CAD build for the part. Positions are in the model's coordinates, mm. A direction names the side the tool comes from. Give positions to 0.01 mm unless a question says otherwise; leave off trailing zeros. Order: outer loops, then holes, each group sorted by start corner. A loop starts at its lowest first (then second) coordinate and runs counter-clockwise, first axis right, second up.
```python
from build123d import *

# Parameters (mm, degrees)
BOSS_EXTRUDE1_DEPTH           = 45
SKETCH3_W                     = 30
SKETCH3_H                     = 40
CUT_EXTRUDE1_DEPTH            = 88.304481557
SKETCH4_W                     = 32
SKETCH4_H                     = 32
SKETCH4_W_2                   = 20.5
SKETCH4_H_2                   = 20.5
BOSS_EXTRUDE2_DEPTH           = 35
SKETCH6_W                     = 5
SKETCH6_H                     = 5
CUT_EXTRUDE4_DEPTH            = 35
RIB1_REACH                    = 87.394
SKETCH9_WALL_W                = 221.994100462
SKETCH9_WALL_H                = 2
LPATTERN1_COUNT               = 2
LPATTERN1_PITCH               = 20
RIB6_REACH                    = 100.659
SKETCH14_WALL_W               = 234.916193708
SKETCH14_WALL_H               = 2
RIB7_START                    = -2
RIB7_DEPTH                    = 2
FILLET2_R                     = 5
FILLET3_R                     = 5
RIB10_REACH                   = 92.525
SKETCH17_WALL_W               = 226.71130823
SKETCH17_WALL_H               = 2
RIB11_REACH                   = 92.525
SKETCH18_WALL_W               = 226.71130823
SKETCH18_WALL_H               = 2
FILLET4_R                     = 10
LPATTERN2_COUNT               = 2
LPATTERN2_PITCH               = 43
FILLET4_OF_LPATTERN2_R        = 10
M5_CLEARANCE_HOLE2_AT_2_COUNT = 2
M5_CLEARANCE_HOLE2_AT_2_PITCH = 15
M2_5_CLEARANCE_HOLE1_D        = 2.9
FILLET5_R                     = 2.5
SKETCH4_4_R                   = 2.5
BOSS_EXTRUDE4_DEPTH           = 8
CIRPATTERN1_COUNT             = 4


# Read off the part's stored shape, not the designer's step: Rib7
with BuildPart() as part:
    # Sketch2 → Boss-Extrude1 (new body)
    with BuildSketch(Plane.XY):
        Polygon((-53.5125, -22.5), (17.8375, -22.5), (17.8375, -17.5), (-8.5125, -17.5), (-8.5125, 22.5), (-13.5125, 22.5), (-13.5125, -17.5), (-48.5125, -17.5), (-48.5125, 22.5), (-53.5125, 22.5), align=None)
    extrude(amount=BOSS_EXTRUDE1_DEPTH)

    # Sketch3 → Cut-Extrude1 (cut, through all)
    with BuildSketch(Plane(origin=(-53.5125, 0, 0), x_dir=(0, 0, -1), z_dir=(1, 0, 0))):
        with Locations((-22.5, 2.5)):
            Rectangle(SKETCH3_W, SKETCH3_H)
    extrude(amount=CUT_EXTRUDE1_DEPTH, mode=Mode.SUBTRACT)

    # Sketch4 → Boss-Extrude2 (add)
    with BuildSketch(Plane.XZ.offset(22.5)):
        with Locations((1.8375, 22.5)):
            Rectangle(SKETCH4_W, SKETCH4_H)
        with Locations((1.8375, 22.5)):
            Rectangle(SKETCH4_W_2, SKETCH4_H_2, mode=Mode.SUBTRACT)
    extrude(amount=BOSS_EXTRUDE2_DEPTH)

    # Sketch6 → Cut-Extrude4 (cut)
    with BuildSketch(Plane(origin=(0, -57.5, 0), x_dir=(-1, 0, 0), z_dir=(0, -1, 0))):
        with Locations((11.6625, -36)):
            Rectangle(SKETCH6_W, SKETCH6_H)
        with Locations((-15.3375, -36)):
            Rectangle(SKETCH6_W, SKETCH6_H)
        with Locations((-15.3375, -9)):
            Rectangle(SKETCH6_W, SKETCH6_H)
        with Locations((11.6625, -9)):
            Rectangle(SKETCH6_W, SKETCH6_H)
    extrude(amount=-CUT_EXTRUDE4_DEPTH, mode=Mode.SUBTRACT)

    # Sketch9 wall → Rib1 (add, up to next)
    with BuildSketch(Plane(origin=(-31.45625, -40, 33.5), x_dir=(-0.70290285213, 0.7112858641, 0), z_dir=(-0.7112858641, -0.70290285213, 0)), mode=Mode.PRIVATE) as rib1_sk1:
        with Locations((0, 1)):
            Rectangle(SKETCH9_WALL_W, SKETCH9_WALL_H)
    rib1_tool1 = extrude(rib1_sk1.sketch, amount=-RIB1_REACH, mode=Mode.PRIVATE) - part.part
    rib1 = rib1_tool1.solids().sort_by_distance((-31.45625, -40, 33.5))[0]
    add(rib1)

    # LPattern1: Rib1 ×2
    with Locations(*[(0, 0, -i * LPATTERN1_PITCH) for i in range(1, LPATTERN1_COUNT)]):
        add(rib1)

    # Sketch14 wall → Rib6 (add, up to next)
    with BuildSketch(Plane(origin=(12.8375, -40, 3.25), x_dir=(0, 0.983188736076, -0.182592193843), z_dir=(0, 0.182592193843, 0.983188736076)), mode=Mode.PRIVATE) as rib6_sk1:
        with Locations((0, 1)):
            Rectangle(SKETCH14_WALL_W, SKETCH14_WALL_H)
    rib6_tool1 = extrude(rib6_sk1.sketch, amount=RIB6_REACH, mode=Mode.PRIVATE) - part.part
    rib6 = rib6_tool1.solids().sort_by_distance((12.8375, -40, 3.25))[0]
    add(rib6)

    # Rib7 outline → Rib7 (add)
    with BuildSketch(Plane.ZY.offset(9.1625).offset(RIB7_START)):
        Polygon((0, -22.5), (6.5, -57.5), (6.5, -22.5), align=None)
    rib7 = extrude(amount=RIB7_DEPTH)

    # Fillet2
    fillet2_edges = [part.edges().sort_by_distance(p)[0] for p in [
        (1.8375, -22.5, 38.5),
        (-14.1625, -22.5, 22.5),
        (1.8375, -22.5, 6.5),
    ]]
    fillet(fillet2_edges, radius=FILLET2_R)

    # Fillet3
    fillet3_edges = [part.edges().sort_by_distance(p)[0] for p in [
        (-8.5125, -17.5, 41.25),
        (-8.5125, -17.5, 3.75),
    ]]
    fillet(fillet3_edges, radius=FILLET3_R)

    # Sketch17 wall → Rib10 (add, up to next)
    with BuildSketch(Plane(origin=(-39.7625, 2.5, 45), x_dir=(0.40081883402, -0.916157334902, 0), z_dir=(0.916157334902, 0.40081883402, 0)), mode=Mode.PRIVATE) as rib10_sk1:
        with Locations((0, 1)):
            Rectangle(SKETCH17_WALL_W, SKETCH17_WALL_H)
    rib10_tool1 = extrude(rib10_sk1.sketch, amount=-RIB10_REACH, mode=Mode.PRIVATE) - part.part
    rib10 = rib10_tool1.solids().sort_by_distance((-39.7625, 2.5, 45))[0]
    add(rib10)

    # Sketch18 wall → Rib11 (add, up to next)
    with BuildSketch(Plane(origin=(-22.2625, 2.5, 45), x_dir=(0.40081883402, 0.916157334902, 0), z_dir=(-0.916157334902, 0.40081883402, 0)), mode=Mode.PRIVATE) as rib11_sk1:
        with Locations((0, 1)):
            Rectangle(SKETCH18_WALL_W, SKETCH18_WALL_H)
    rib11_tool1 = extrude(rib11_sk1.sketch, amount=-RIB11_REACH, mode=Mode.PRIVATE) - part.part
    rib11 = rib11_tool1.solids().sort_by_distance((-22.2625, 2.5, 45))[0]
    add(rib11)

    # Fillet4
    # the kernel refuses this fillet: 10 mm, written as the material it adds along each edge
    with BuildSketch(Plane(origin=(-31.0125, -17.5, 45), x_dir=(-0.4008188340200226, 0.9161573349020513, 0), z_dir=(0, 0, -1))) as fillet4_piece_1:
        with BuildLine():
            CenterArc((FILLET4_R * 2.28571428571, FILLET4_R), FILLET4_R, 137.258755461, 132.741244539)
            Line((FILLET4_R * 1.55128805621, FILLET4_R * 1.67868852459), (0, 0))
            Line((0, 0), (FILLET4_R * 2.28571428571, 0))
        make_face()
    extrude(amount=2)

    # LPattern2: Rib10, Rib11 ×2
    with Locations(*[(0, 0, -i * LPATTERN2_PITCH) for i in range(1, LPATTERN2_COUNT)]):
        add(rib10)
        add(rib11)

    # Fillet4 of LPattern2
    # the kernel refuses this fillet: 10 mm, written as the material it adds along each edge
    with BuildSketch(Plane(origin=(-31.0125, -17.5, 59.142857143), x_dir=(-0.4008188340200225, 0.9161573349020515, 0), z_dir=(0, 0, -1))) as fillet4_of_lpattern2_piece_1_section:
        with BuildLine():
            CenterArc((FILLET4_OF_LPATTERN2_R * 2.28571428571, FILLET4_OF_LPATTERN2_R), FILLET4_OF_LPATTERN2_R, 137.258755461, 132.741244539)
            Line((FILLET4_OF_LPATTERN2_R * 1.5512880562, FILLET4_OF_LPATTERN2_R * 1.67868852459), (0, 0))
            Line((0, 0), (FILLET4_OF_LPATTERN2_R * 2.28571428571, 0))
        make_face()
    fillet4_of_lpattern2_piece_1 = extrude(amount=59.142857143, mode=Mode.PRIVATE)
    fillet4_of_lpattern2_piece_1 = split(fillet4_of_lpattern2_piece_1, bisect_by=Plane(origin=(-31.0125, -6.732617491, 43), z_dir=(0, 0, 1)), keep=Keep.TOP, mode=Mode.PRIVATE)
    fillet4_of_lpattern2_piece_1 = split(fillet4_of_lpattern2_piece_1, bisect_by=Plane(origin=(-31.0125, -6.732617491, 45), z_dir=(0, 0, -1)), keep=Keep.TOP, mode=Mode.PRIVATE)
    add(fillet4_of_lpattern2_piece_1)
    with BuildSketch(Plane(origin=(-31.0125, -17.5, 2), x_dir=(-0.4008188340200226, 0.9161573349020513, 0), z_dir=(0, 0, -1))) as fillet4_of_lpattern2_piece_2:
        with BuildLine():
            CenterArc((FILLET4_OF_LPATTERN2_R * 2.28571428571, FILLET4_OF_LPATTERN2_R), FILLET4_OF_LPATTERN2_R, 137.258755461, 132.741244539)
            Line((FILLET4_OF_LPATTERN2_R * 1.55128805621, FILLET4_OF_LPATTERN2_R * 1.67868852459), (0, 0))
            Line((0, 0), (FILLET4_OF_LPATTERN2_R * 2.28571428571, 0))
        make_face()
    extrude(amount=2)

    # Sketch22 → M5 Clearance Hole2 (revolve, cut)
    with BuildSketch(Plane(origin=(1.8375, -32.5, 38.5), x_dir=(0, -1, 0), z_dir=(1, 0, 0))):
        Polygon((0, 0), (0, 7.652366702), (2.75, 6), (2.75, 0), align=None)
    m5_clearance_hole2 = revolve(axis=Axis((1.8375, -32.5, 44.85), (0, 0, -1)), mode=Mode.SUBTRACT)

    # M5 Clearance Hole2 at 2: M5 Clearance Hole2 ×2
    with Locations(*[(0, -i * M5_CLEARANCE_HOLE2_AT_2_PITCH, 0) for i in range(1, M5_CLEARANCE_HOLE2_AT_2_COUNT)]):
        add(m5_clearance_hole2, mode=Mode.SUBTRACT)

    # M2.5 Clearance Hole1 (through all)
    with Locations(Plane.ZY.offset(53.5125)):
        with Locations((5.2, 15.5), (39.8, 15.5), (39.8, -6.5), (5.2, -6.5)):
            Hole(M2_5_CLEARANCE_HOLE1_D / 2)

    # Fillet5
    fillet5_edges = [part.edges().sort_by_distance(p)[0] for p in [
        (-9.1625, -40, 11.5),
        (12.8375, -40, 11.5),
        (12.8375, -40, 33.5),
        (-9.1625, -40, 33.5),
    ]]
    fillet(fillet5_edges, radius=FILLET5_R)

    # Sketch4<4> → Boss-Extrude4 (add)
    with BuildSketch(Plane.XZ.offset(22.5)):
        with Locations(Location((1.8375, 22.5, 0), (0, 0, 180))):
            Circle(SKETCH4_4_R)
    extrude(amount=BOSS_EXTRUDE4_DEPTH)

    # CirPattern1: M5 Clearance Hole2 ×4 about axis
    cirpattern1_axis = Axis((1.8375, -30.5, 22.5), (0, -1, 0))
    for i in range(1, CIRPATTERN1_COUNT):
        add(m5_clearance_hole2.rotate(cirpattern1_axis, i * 360 / CIRPATTERN1_COUNT), mode=Mode.SUBTRACT)

    # CirPattern1 copy 1 sketch → CirPattern1 copy 1 (revolve, cut)
    with BuildSketch(Plane(origin=(-14.1625, -47.5, 22.5), x_dir=(0, -1, 0), z_dir=(0, 0, 1))):
        Polygon((0, 0), (0, 7.652366702), (2.75, 6), (2.75, 0), align=None)
    revolve(axis=Axis((-20.5125, -47.5, 22.5), (1, 0, 0)), mode=Mode.SUBTRACT)

    # CirPattern1 copy 2 sketch → CirPattern1 copy 2 (revolve, cut)
    with BuildSketch(Plane(origin=(1.8375, -47.5, 6.5), x_dir=(0, -1, 0), z_dir=(-1, 0, 0))):
        Polygon((0, 0), (0, 7.652366702), (2.75, 6), (2.75, 0), align=None)
    revolve(axis=Axis((1.8375, -47.5, 0.15), (0, 0, 1)), mode=Mode.SUBTRACT)

    # CirPattern1 copy 3 sketch → CirPattern1 copy 3 (revolve, cut)
    with BuildSketch(Plane(origin=(17.8375, -47.5, 22.5), x_dir=(0, -1, 0), z_dir=(0, 0, -1))):
        Polygon((0, 0), (0, 7.652366702), (2.75, 6), (2.75, 0), align=None)
    revolve(axis=Axis((24.1875, -47.5, 22.5), (-1, 0, 0)), mode=Mode.SUBTRACT)

    # Mirror1: Rib6, Rib7 across plane
    add(rib6.mirror(Plane.XY.offset(22.5)))
    add(rib7.mirror(Plane.XY.offset(22.5)))


solid = part.part
```
Item 1: Two-plate mould, pull along X, no slides. Class faces 1 (the face through (12.838, -36, 39)), 2 (the face through (-11.328, -44.753, 22.379)), 3 (the face through (-17.74, 12.84, 0.99)), 4 (the face through (-9.162, -36, 40)): released by +X, released by -X, zero draft, split by the parting line, or undercut.
Item 2: Wall check: L1, parallel to Y at x = -10.3, z = 39.8; L2, parallel to X at y = -45, z = 19; L3, parallel to Z at x = -30, y = -17. Give the ranges that are in metal, low to high.
Item 3: Drop flat-ended pins along their axis: pin 1 Ø3 at (x, y) = (17, -47.5) entering from +Z; pin 2 Ø6 at (x, z) = (4.5, 17.5) entering from -Y; pin 3 Ø20 at (x, y) = (6, -49) entering from +Z. Give the stop position or say it passes through.
Item 4: Slice it at D-D (x = -16). Give the cut face in (y, z), and give its area (3 significant figures).
Item 5: Tool access for faces 5 (the face through (-11, 2, 7.5)), 6 (the face through (-7.162, -32, 5)), 7 (the face through (-15.666, -23.926, 22.626)): list every direction of +Z, -Z, +X, -X, +Y, -Y with a clear straight run to the whole face (end or side of a thin tool).
Item 6: Slice it at C-C (y = 9.5). Give the cut face in (x, z) (1 decimal), and give its area (4 significant figures).
Item 7: Slice it at A-A (y = -25.5). State how many separate pieces and enclosed holes the cut face has, and give its area (3 significant figures).
A:
1. face 1: released by +X
1. face 2: zero draft
1. face 3: undercut
1. face 4: released by -X
2. L1: y = -22.5 to -7.95, -5.05 to 14.05, 16.95 to 22.5
2. L2: x = -14.16 to -8.41, 12.09 to 17.84
2. L3: z = 0 to 2, 43 to 45
3. pin 1: stops at z = 33.5
3. pin 2: stops at y = -22.5
3. pin 3: stops at z = 41.7
4. outline: (-55.64, 11.5) - (-22.5, 11.5) - (-22.5, 0) - (16.81, 0) - (16.81, 2) - (-17.5, 2) - (-17.5, 43) - (16.81, 43) - (16.81, 45) - (-22.5, 45) - (-22.5, 33.5) - (-55.64, 33.5) - (-55.64, 31.5) - (-23.63, 31.5) - (-23.63, 13.5) - (-55.64, 13.5) - close
4. area: 515 mm2
5. face 5: +X, -X, +Y
5. face 6: -Z, -Y
5. face 7: -X, -Y
6. outline: (-53.5, 0) - (-42.8, 0) - (-42.8, 2) - (-48.5, 2) - (-48.5, 7.5) - (-53.5, 7.5) - close; (-53.5, 37.5) - (-48.5, 37.5) - (-48.5, 43) - (-42.8, 43) - (-42.8, 45) - (-53.5, 45) - close; (-19.2, 0) - (-8.5, 0) - (-8.5, 7.5) - (-13.5, 7.5) - (-13.5, 2) - (-19.2, 2) - close; (-19.2, 43) - (-13.5, 43) - (-13.5, 37.5) - (-8.5, 37.5) - (-8.5, 45) - (-19.2, 45) - close
6. area: 195.5 mm2
7. separate pieces: 2
7. enclosed holes: 1
7. area: 725 mm2
